The model under review builds one solid part; all positions refer to its coordinate system, in mm. A direction names the side the tool comes from. Give positions to 0.01 mm unless a question says otherwise; leave off trailing zeros. Write each loop counter-clockwise with the first axis right and the second up, starting at its lowest first coordinate (ties: lowest second). Pieces come first, ordered by that corner, then holes. Notation, with made-up numbers: M 62,-35 L 85,-35 A18 cw 85,-29 Z; hole C -8.5,-17.5 d11. An arc over 180 degrees is marked long. Write item = value, one per line. Start each with the question number.
Autodesk Inventor part; units mm, degrees
ref_plane "YZ Plane" through (0, 0, 0) normal (1, 0, 0) x (0, 1, 0)
ref_plane "XZ Plane" through (0, 0, 0) normal (0, 1, 0) x (-1, 0, 0)
ref_plane "XY Plane" through (0, 0, 0) normal (0, 0, 1) x (1, 0, 0)
sketch "Sketch1" plane through (0, 0, 0) normal (0, 1, 0) x (-1, 0, 0)
  line L0 (0, 0) -> (30, 0)
  line L1 (30, 0) -> (30, -30)
  line L2 (30, -30) -> (0, -30)
  line L3 (0, -30) -> (0, 0)
  line L4 (28, -2) -> (2, -2)
  line L5 (2, -2) -> (2, -28)
  line L6 (2, -28) -> (28, -28)
  line L7 (28, -28) -> (28, -2)
  line L8 (28, -2) -> (2, -28) construction
  line L9 (2, -2) -> (28, -28) construction
  circle A0 centre (28, -2) radius 1.5
  circle A1 centre (28, -28) radius 1.5
  circle A2 centre (2, -2) radius 1.5
  circle A3 centre (2, -28) radius 1.5
  point P0 (15, -15)
  dimension "d0" = 30
  dimension "d1" = 30
  dimension "d2" = 26
  dimension "d3" = 26
  dimension "d4" = 3
  dimension "d7" = 26
  dimension "d10" = 26
extrude "Extrusion1" add sketch "Sketch1" against normal blind 3.175 contours L0 L1 L2 L3 | A2 L5 L4 | L4 L5 A2 | L4 A0 L7 A1 L6 A3 L5 A2 | A0 L7 L4 | L4 L7 A0 | A3 L6 L5 | L5 L6 A3 | A1 L6 L7 | L7 L6 A1
extrude "Extrusion2" add sketch "Sketch1" along normal blind 6.35 contours A2 L5 L4 | L4 L5 A2 | A0 L7 L4 | L4 L7 A0 | A3 L6 L5 | L5 L6 A3 | A1 L6 L7 | L7 L6 A1
sketch "Sketch2" plane through (0, 0, 0) normal (1, 0, 0) x (0, 0, -1)
  line L0 (0, 0) -> (0, -3.175)
  line L1 (0, 0) -> (30, 0)
  line L2 (0, -3.175) -> (30, -3.175)
  line L3 (30, -3.175) -> (30, 0)
  line L4 (30, 0) -> (0, 0)
  line L5 (0, 0) -> (0, -3.175)
extrude "Extrusion3" add sketch "Sketch2" along normal blind 6.35
sketch "Sketch3" plane through (0, 0, 0) normal (0, 1, 0) x (1, 0, 0)
  line L0 (6.35, 0) -> (6.35, 30)
  line L1 (-30, 30) -> (6.35, 30)
  line L2 (6.35, 0) -> (3.175, 0)
  line L3 (3.175, 0) -> (3.175, 30)
  line L4 (3.175, 30) -> (6.35, 30)
  line L5 (6.35, 30) -> (6.35, 0)
  point P0 (0, 0)
  dimension "d19" = 3.175
extrude "Extrusion4" add sketch "Sketch3" along normal blind 13.175
sketch "Sketch4" plane through (6.35, 0, 0) normal (1, 0, 0) x (0, 0, -1)
  line L0 (30, 13.175) -> (0, 13.175)
  line L1 (30, 0) -> (30, 13.175)
  line L2 (0, 13.175) -> (30, 13.175)
  line L3 (15, 13.175) -> (15, 11.5875)
  line L4 (15, 11.5875) -> (27.7, 11.5875)
  line L5 (27.7, 11.5875) -> (2.3, 11.5875)
  circle A0 centre (2.3, 11.5875) radius 1.5875
  circle A1 centre (27.7, 11.5875) radius 1.5875
  line L6 (4.7076, 10) -> (25.2924, 10)
  line L7 (25.2924, 10) -> (25.2924, 13.175)
  line L8 (25.2924, 13.175) -> (4.7076, 13.175)
  line L9 (4.7076, 13.175) -> (4.7076, 10)
  line L10 (4.7076, 10) -> (25.2924, 13.175) construction
  line L11 (25.2924, 10) -> (4.7076, 13.175) construction
  line L12 (8.65, 6.825) -> (21.35, 6.825)
  line L13 (21.35, 6.825) -> (21.35, 13.175)
  line L14 (21.35, 13.175) -> (8.65, 13.175)
  line L15 (8.65, 13.175) -> (8.65, 6.825)
  line L16 (8.65, 6.825) -> (21.35, 13.175) construction
  line L17 (21.35, 6.825) -> (8.65, 13.175) construction
  point P0 (0, 0)
  point P1 (15, 10)
  point P2 (21.35, 10)
  point P3 (8.65, 10)
  dimension "d22" = 1.5875
  dimension "d23" = 12.7
  dimension "d24" = 90
  dimension "d25" = 25.4
  dimension "d26" = 3.175
  dimension "d27" = 3.175
extrude "Extrusion5" add sketch "Sketch4" along normal blind 31.75 contours A1 | A0
extrude "Extrusion6" cut sketch "Sketch4" against normal blind 3.175 contours L7 L4 L13 L0 | L13 L4 L3 L0 | L7 L6 L13 L4 | L3 L5 L15 L0 | L13 L6 L15 L5 L4 | L15 L5 L9 L0 | L13 L12 L15 L6 | L15 L6 L9 L5
mirror "Mirror1" about plane through (38.1, 11.5875, -27.7) normal (1, 0, 0) of "Extrusion1", "Extrusion2", "Extrusion3", "Extrusion4", "Extrusion5", "Extrusion6"
properties part number "CDSAXS-Capillary-Frame-For2Sensors"
Item 1: Clearance check with flat-ended pins moving along their axes: P1, Ø12, axis at x = 23, z = -9, coming from the +Y side; P2, Ø6, axis at x = 42.5, z = -21, coming from the +Y side; P3, Ø3.5, axis at x = 5, z = -23.5, coming from the +Y side; P4, Ø4, axis at y = 8.5, z = -9, coming from the +X side (3 decimals). State where each tip first meets the part, or that it passes through.
Item 2: For faces 4 (the flat face through (-28, 6.35, -2)), 5 (the flat face through (3.175, 5, -15)), 6 (the cylindrical face through (78.005, 3.131, -26.513)), 7 (the flat face through (71, 10, -7)), list the 3-axis set-ups (+Z, -Z, +X, -X, +Y, -Y) from which the entire face can be reached by the end or side of a thin tool; tool diameter is ignored.
Item 3: We need section D-D, the plane x = 46. Write out the cut boundary in (y, z) (1 decimal), and give its area (3 significant figures).
Item 4: We need section A-A, the plane y = 3.5. Give the number of separate pieces and of enclosed holes in the cut face, and give its area (3 significant figures).
Item 5: To check wall thickness, follow probe 1 along X at (y, z) = (-2, -12.5); probe 2 along X at (y, z) = (1, -24.25) (3 decimals); probe 3 along Y at (x, z) = (-14, -28) (3 decimals). State the ranges of each line that lie inside material, in increasing order. Write a range as [from, to].
Item 6: We need section B-B, the plane z = -19. Write out the cut boundary in (x, y) (3 decimals).
Item 7: We need section C-C, the plane x = -2. Write out the cut boundary in (y, z) (3 decimals).
Item 8: The part is to be moulded in two halves that separate along Z. For faces 1 (the flat face through (84.1, -0.5, 0)), 2 (the flat face through (5, 6.825, -15)), 3 (the flat face through (88, -3.175, -15)), say which applies: released by +Z, released by -Z, zero draft, split by the parting line, or undercut.
Worked out:
q1.P1 = 13.01
q1.P2 = through
q1.P3 = 10
q1.P4 = 73.025
q2.face_4 = +Z, -Z, -X, +Y
q2.face_5 = +Z, -Z, +Y
q2.face_6 = +Y
q2.face_7 = +X, -X, +Y
q3.outline = C 11.6,-27.7 d3.2; C 11.6,-2.3 d3.2
q3.area = 15.8 mm²
q4.separate_pieces = 10
q4.enclosed_holes = 0
q4.area = 247 mm²
q5.probe_1 = [-30, 6.35], [69.85, 106.2]
q5.probe_2 = [3.175, 6.35], [69.85, 73.025]
q5.probe_3 = [-3.175, 0]
q6.outline = M -30,-3.175 L 6.35,-3.175 L 6.35,6.825 L 3.175,6.825 L 3.175,0 L -30,0 Z; M 69.85,-3.175 L 106.2,-3.175 L 106.2,0 L 73.025,0 L 73.025,6.825 L 69.85,6.825 Z
q7.outline = M -3.175,-30 L 0,-30 L 0,-29.5 L 6.35,-29.5 L 6.35,-26.5 L 0,-26.5 L 0,-3.5 L 6.35,-3.5 L 6.35,-0.5 L 0,-0.5 L 0,0 L -3.175,0 Z
q8.face_1 = released by +Z
q8.face_2 = undercut
q8.face_3 = zero draft
